from build123d import *

# Parameters (mm, degrees)
BOX008_W        = 1828.8
BOX008_H        = 38.1
BOX008_DEPTH    = 88.9
POCKET005_DEPTH = 38.1010000002


with BuildPart() as pocket005:
    # Box008 → Box008 (new body)
    with BuildSketch(Plane(origin=(-152.4, -38.1, 457.2), x_dir=(1, 0, 0), z_dir=(0, 0, 1))):
        with Locations((914.4, 19.05)):
            Rectangle(BOX008_W, BOX008_H)
    extrude(amount=BOX008_DEPTH)

    # Sketch005 → Pocket005 (cut, through all)
    with BuildSketch(Plane(origin=(-152.4, -38.1, 457.2), x_dir=(1, 0, 0), z_dir=(0, -1, 0))):
        Polygon((190.5, 44.45), (152.4, 44.45), (152.4, 88.9), (0, 88.9), (0, 0), (190.5, 0), align=None)
        Polygon((1638.3, 44.45), (1676.4, 44.45), (1676.4, 88.9), (1828.8, 88.9), (1828.8, 0), (1638.3, 0), align=None)
    extrude(amount=-POCKET005_DEPTH, mode=Mode.SUBTRACT)


with BuildPart() as southfloorbeam:
    # Part__Mirroring003: instance of Pocket005
    add(pocket005.part.mirror(Plane(origin=(0, 762, 0), x_dir=(1, 0, 0), z_dir=(0, 1, 0))))


solid = southfloorbeam.part
Check sheet for the modelled part. Datum: model origin and axes. Units: mm. A direction names the side the tool comes from. Give positions to 0.01 mm unless a question says otherwise; leave off trailing zeros. Loops run counter-clockwise (first coordinate to the right, second up) from the corner with the lowest first, then second, coordinate; pieces in that order, holes last. Notation, with made-up numbers: M 59.25,65 L 95.25,65 A15 ccw 95.25,82 Z; hole C 39,60.25 d5. An arc over 180 degrees is marked long. Answer as a JSON object with one key per item and string values. Group by question number.
Q1. Access from +Z, -Z, +X, -X, +Y, -Y to the whole of each face (thin tool, end or side, straight path). Record for faces 1 (the flat face through (1505, 1543, 501.65)), 2 (the flat face through (38.1, 1543, 479)), 3 (the flat face through (751, 1543, 546.1)).
Q2. Cross-section at B-B on z = 480. Record the cut outline in (x, y), then the cut area to 3 significant figures.
Q3. Material ranges on line 1 along X through (y, z) = (1538.5, 491.5), recorded low to high. Write a range as [from, to].
Q4. Go/stop test with flat-tipped pins: P1, Ø5, axis at y = 1535.5, z = 483, coming from the +X side; P2, Ø11.5, axis at x = 1501, y = 1550, coming from the -Z side; P3, Ø8, axis at y = 1545.5, z = 517.5, coming from the -X side. Record where each tip stops, or that it passes through.
Q5. Cross-section at A-A on y = 1545. Record the cut outline in (x, z), then the cut area to 3 significant figures.
Evaluation:
{
 "1": {"face 1": "-Z, +X, +Y, -Y", "face 2": "-Z, -X, +Y, -Y", "face 3": "+Z, +X, -X, +Y, -Y"},
 "2": {"outline": "M 38.1,1524 L 1485.9,1524 L 1485.9,1562.1 L 38.1,1562.1 Z", "area": "55,200 mm2"},
 "3": {"line 1": "x = [38.1, 1485.9]"},
 "4": {"P1": "stops at x = 1485.9", "P2": "stops at z = 501.65", "P3": "stops at x = 0"},
 "5": {"outline": "M 0,501.65 L 38.1,501.65 L 38.1,457.2 L 1485.9,457.2 L 1485.9,501.65 L 1524,501.65 L 1524,546.1 L 0,546.1 Z", "area": "132,000 mm2"}
}
